Input: part model. Units: mm. Frame: model coordinates. Round coordinates to 2 decimals unless told otherwise and drop trailing zeros. Loops run counter-clockwise (first coordinate to the right, second up) from the corner with the lowest first, then second, coordinate; pieces in that order, holes last. Notation, with made-up numbers: M 11,82.5 L 32,82.5 A16 cw 32,106.5 Z; hole C -30,8.5 d9. An arc over 180 degrees is marked long. Put each result on its own line as item: value. Start each with the question number.
1) Section A-A on z = -3.5. Output: boundary loops of the cut face in (x, y), plus the area to 3 significant figures.
2) Pin query (flat end, axial travel): pin 1 (4 mm diameter, centred on x = 19.5, z = 1.5, fed in from -Y); pin 2 (4 mm diameter, centred on x = 1.5, z = -12.5, fed in from -Y); pin 3 (12 mm diameter, centred on x = -11, z = 6, fed in from -Y). Return the tip coordinate at first contact, or that it passes through.
3) Line query: probe 1 along X at (y, z) = (22, -22); probe 2 along X at (y, z) = (13, 0.5); probe 3 along Y at (x, z) = (23.5, -14). Output: solid intervals per line, ascending.
from build123d import *

# Parameters (mm, degrees)
F3_R = 5.08
F4_R = 5.08


with BuildPart() as f2:
    # F0 (on Front) → F2 (revolve)
    with BuildSketch(Plane.XZ):
        with BuildLine():
            Line((30.48, 18.0614531664), (0, 18.0614531664))
            Line((0, 18.0614531664), (0, -26.3885468336))
            Line((0, -26.3885468336), (43.688, -26.3885468336))
            Line((43.688, -26.3885468336), (43.688, 6.6314531664))
            ThreePointArc((43.688, 6.6314531664), (34.8601557432, 9.7766775807), (30.48, 18.0614531664))
        make_face()
    revolve(axis=Axis((0, 0, -49.3586864322), (0, 0, -1)))

    # F3
    f3_edges = [f2.edges().sort_by_distance(p)[0] for p in [
        (-30.48, 0, 18.061453),
    ]]
    fillet(f3_edges, radius=F3_R)

    # F4
    f4_edges = [f2.edges().sort_by_distance(p)[0] for p in [
        (-43.688, 0, 6.631453),
    ]]
    fillet(f4_edges, radius=F4_R)


solid = f2.part
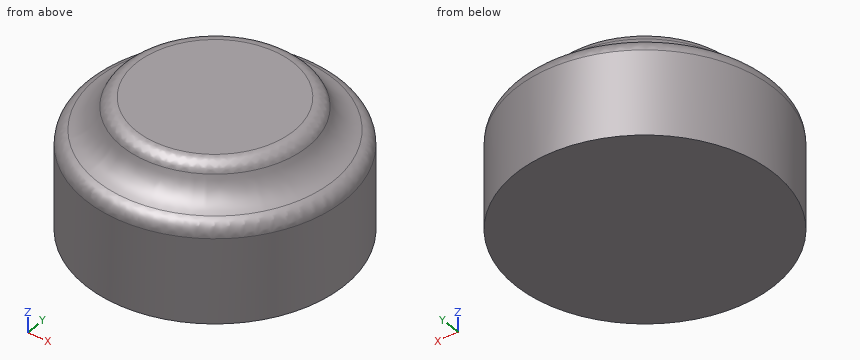
Geometry results:
1. outline: C 0,0 d87.38
1. area: 6,000 mm²
2. pin 1: stops at y = -40.03
2. pin 2: stops at y = -43.69
2. pin 3: stops at y = -43.25
3. probe 1: x = -37.74 to 37.74
3. probe 2: x = -41.71 to 41.71
3. probe 3: y = -36.83 to 36.83
